The drawing under review shows one solid part. Ordinate dimensions are in mm from its lowest x, y, z. Round coordinates to 2 decimals unless told otherwise and drop trailing zeros. Order: outer loops, then holes, each group sorted by start corner. A loop starts at its lowest first (then second) coordinate and runs counter-clockwise, first axis right, second up. Notation, with made-up numbers: M 45,12.25 L 60,12.25 A16 ccw 60,17.25 Z; hole C 1.25,-18 d11. An arc over 180 degrees is marked long. Write item = value, one per line. Start each with the question number.
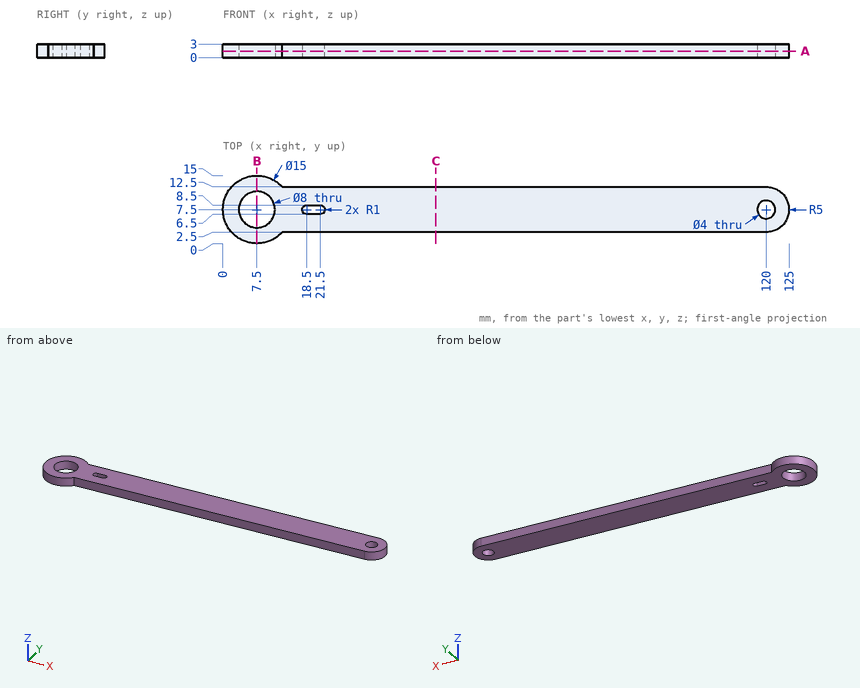
(1) Consider section B-B, the plane x = 7.5. Write out the cut boundary in (y, z), then the cut area to 3 significant figures.
(2) Consider section C-C, the plane x = 47. Write out the cut boundary in (y, z).
(3) Consider section A-A, the plane z = 1.4. Write out the cut boundary in (x, y), then the cut area to 3 significant figures.
(4) Insertion check: pin 1 (2 mm diameter, centred on x = 34.5, y = 8, fed in from -Z); pin 2 (1 mm diameter, centred on y = 6.5, z = 2, fed in from +X). Each pin has a flat end and moves straight along its axis. Give the tip position at first contact, or say it passes through.
(5) For line 1 along Y through (x, z) = (7.5, 1.15); line 2 along Y through (x, z) = (120, 1.7); line 3 along X through (y, z) = (6.75, 2.4), list the stretches that pass through material, from the lowest coordinate up. Write a range as [from, to].
Completed:
q1.outline = M 0,0 L 3.5,0 L 3.5,3 L 0,3 Z; M 11.5,0 L 15,0 L 15,3 L 11.5,3 Z
q1.area = 21.0 mm2
q2.outline = M 2.5,0 L 12.5,0 L 12.5,3 L 2.5,3 Z
q3.outline = M 13.09,2.5 L 120,2.5 A5 ccw 120,12.5 L 13.09,12.5 A7.5 ccw long Z; hole C 7.5,7.5 d8; hole M 18.5,6.5 L 21.5,6.5 A1 ccw 21.5,8.5 L 18.5,8.5 A1 ccw Z; hole C 120,7.5 d4
q3.area = 1,200 mm2
q4.pin_1 = 0
q4.pin_2 = 124.97
q5.line_1 = [0, 3.5], [11.5, 15]
q5.line_2 = [2.5, 5.5], [9.5, 12.5]
q5.line_3 = [0.04, 3.57], [11.43, 17.84], [22.16, 118.15], [121.85, 124.94]
